Check sheet for the modelled part. Datum: model origin and axes. Units: mm. A direction names the side the tool comes from. Round coordinates to 2 decimals unless told otherwise and drop trailing zeros. Write each loop counter-clockwise with the first axis right and the second up, starting at its lowest first coordinate (ties: lowest second). Pieces come first, ordered by that corner, then holes.
Item 1: Material ranges on line 1 (X direction, y = 0, z = 4.25); line 2 (Y direction, x = -12.7, z = -0.45), recorded low to high.
Item 2: Tool access check on faces 5 (the flat face through (-27, -9.525, 18)), 6 (the flat face through (-17.368, 0, 10)), 7 (the flat face through (-27, 9.525, 18)), 8 (the cylindrical face through (13.655, -18.808, 18.716)), 9 (the flat face through (27, 9.525, 18)). Record the directions out of +Z, -Z, +X, -X, +Y, -Y that give a thin tool (end or side, any length) a straight path to the whole face; none if there is none.
Item 3: Cross-section at B-B on x = -14.5. Enter the section's corners in (y, z), plus the area to 3 significant figures.
Item 4: Cross-section at C-C on z = 0. Enter the section's corners in (x, y) (3 decimals), plus the area to 3 significant figures.
Item 5: Go/stop test with flat-tipped pins: pin 1 Ø4.5 at (x, y) = (26.64, 0) entering from +Z; pin 2 Ø5 at (x, y) = (-0.5, -16) entering from +Z; pin 3 Ø6.5 at (y, z) = (5, 6.5) entering from +X; pin 4 Ø8 at (y, z) = (-3, 6.5) entering from -X. Record where each tip stops, or that it passes through.
Item 6: Release check for a two-part mould opening along Y. For faces 1 (the flat face through (27, -9.525, 18)), 2 (the flat face through (0, 20.289, 9)), 3 (the cylindrical face through (11.79, -18.81, 2.54)), 4 (the cylindrical face through (10.684, -1.546, -0.022)) record: +Y half, -Y half, draft (parallel to the pull), parting line (faces both ways), or undercut.
Item 7: Cross-section at A-A on y = 0. Enter the section's corners in (x, z), plus the area to 3 significant figures.
Item 8: Cross-section at D-D on x = -1. Enter the section's corners in (y, z).
from build123d import *

# Parameters (mm, degrees)
SKETCH1_W           = 40.57777
SKETCH1_H           = 40.57777
SKETCH1_R           = 2.54
BOSS_EXTRUDE1_DEPTH = 1.5875
SKETCH3_W           = 40.57777
SKETCH3_H           = 40.57777
SKETCH3_W_2         = 34.73577
SKETCH3_H_2         = 34.73577
BOSS_EXTRUDE2_DEPTH = 18.034
SKETCH4_W           = 12.7
SKETCH4_H           = 19.05
SKETCH4_R           = 2.4892
BOSS_EXTRUDE3_DEPTH = 3.175
FILLET1_R           = 3.175
SKETCH6_W           = 25.4
SKETCH6_H           = 18.034
CUT_EXTRUDE2_DEPTH  = 3.175
FILLET3_R           = 3.175


with BuildPart() as part:
    # Sketch1 → Boss-Extrude1 (new, symmetric)
    with BuildSketch(Plane.XY):
        Rectangle(SKETCH1_W, SKETCH1_H)
        with Locations((-12.7, 0)):
            Circle(SKETCH1_R, mode=Mode.SUBTRACT)
        with Locations((12.7, 0)):
            Circle(SKETCH1_R, mode=Mode.SUBTRACT)
    extrude(amount=BOSS_EXTRUDE1_DEPTH, both=True)

    # Sketch3 → Boss-Extrude2 (add)
    with BuildSketch(Plane.XY.offset(1.5875)):
        Rectangle(SKETCH3_W, SKETCH3_H)
        Rectangle(SKETCH3_W_2, SKETCH3_H_2, mode=Mode.SUBTRACT)
    extrude(amount=BOSS_EXTRUDE2_DEPTH)

    # Sketch4 → Boss-Extrude3 (add)
    # profile 1 of 2: a face of its own
    with BuildSketch(Plane.XY.offset(19.6215)):
        with Locations((-26.638885, 0)):
            Rectangle(SKETCH4_W, SKETCH4_H)
        with Locations((-26.638885, 0)):
            Circle(SKETCH4_R, mode=Mode.SUBTRACT)
    # profile 2 of 2: a face of its own
    with BuildSketch(Plane.XY.offset(19.6215)):
        with Locations((26.638885, 0)):
            Rectangle(SKETCH4_W, SKETCH4_H)
        with Locations((26.638885, 0)):
            Circle(SKETCH4_R, mode=Mode.SUBTRACT)
    extrude(amount=-BOSS_EXTRUDE3_DEPTH)

    # Fillet1
    fillet1_edges = [part.edges().sort_by_distance(p)[0] for p in [
        (-20.288885, 9.525, 18.034),
        (-20.288885, -9.525, 18.034),
        (-32.988885, -9.525, 18.034),
        (-32.988885, 9.525, 18.034),
        (20.288885, -9.525, 18.034),
        (20.288885, 9.525, 18.034),
        (32.988885, 9.525, 18.034),
        (32.988885, -9.525, 18.034),
        (20.288885, -20.288885, 9.017),
        (-20.288885, -20.288885, 9.017),
        (-20.288885, 20.288885, 9.017),
        (20.288885, 20.288885, 9.017),
    ]]
    fillet(fillet1_edges, radius=FILLET1_R)

    # Sketch6 → Cut-Extrude2 (cut)
    with BuildSketch(Plane.XZ.offset(20.288885)):
        with Locations((0, 10.6045)):
            Rectangle(SKETCH6_W, SKETCH6_H)
    extrude(amount=-CUT_EXTRUDE2_DEPTH, mode=Mode.SUBTRACT)

    # Fillet3
    fillet3_edges = [part.edges().sort_by_distance(p)[0] for p in [
        (-12.7, -18.828385, 1.5875),
        (-12.7, -18.828385, 19.6215),
        (12.7, -18.828385, 19.6215),
        (12.7, -18.828385, 1.5875),
    ]]
    fillet(fillet3_edges, radius=FILLET3_R)


solid = part.part
Response values:
1. line 1: x = -20.29 to -17.37, 17.37 to 20.29
1. line 2: y = -20.29 to -2.54, 2.54 to 20.29
2. face 5: +Z, -Z, -X, -Y
2. face 6: +Z
2. face 7: +Z, -Z, -X, +Y
2. face 8: +Z, -Y
2. face 9: +Z, -Z, +X, +Y
3. outline: (-20.29, -1.59) - (-1.79, -1.59) - (-1.79, 1.59) - (-17.37, 1.59) - (-17.37, 19.31) - (-20.29, 19.31) - close; (1.79, -1.59) - (20.29, -1.59) - (20.29, 19.62) - (17.37, 19.62) - (17.37, 1.59) - (1.79, 1.59) - close
3. area: 222 mm2
4. outline: (-20.289, -17.114) arc R3.175 ccw to (-17.114, -20.289) - (17.114, -20.289) arc R3.175 ccw to (20.289, -17.114) - (20.289, 17.114) arc R3.175 ccw to (17.114, 20.289) - (-17.114, 20.289) arc R3.175 ccw to (-20.289, 17.114) - close; hole circle Ø5.08 at (-12.7, 0); hole circle Ø5.08 at (12.7, 0)
4. area: 1,600 mm2
5. pin 1: passes through
5. pin 2: stops at z = 1.59
5. pin 3: stops at x = 20.29
5. pin 4: stops at x = -20.29
6. face 1: -Y half
6. face 2: +Y half
6. face 3: draft
6. face 4: undercut
7. outline: (-32.99, 16.45) - (-29.13, 16.45) - (-29.13, 19.62) - (-32.99, 19.62) - close; (-24.15, 16.45) - (-20.29, 16.45) - (-20.29, -1.59) - (-15.24, -1.59) - (-15.24, 1.59) - (-17.37, 1.59) - (-17.37, 19.62) - (-24.15, 19.62) - close; (-10.16, -1.59) - (10.16, -1.59) - (10.16, 1.59) - (-10.16, 1.59) - close; (15.24, -1.59) - (20.29, -1.59) - (20.29, 16.45) - (24.15, 16.45) - (24.15, 19.62) - (17.37, 19.62) - (17.37, 1.59) - (15.24, 1.59) - close; (29.13, 16.45) - (32.99, 16.45) - (32.99, 19.62) - (29.13, 19.62) - close
7. area: 251 mm2
8. outline: (-20.29, -1.59) - (20.29, -1.59) - (20.29, 19.62) - (17.37, 19.62) - (17.37, 1.59) - (-20.29, 1.59) - close
